Can you work these out from the model? Positions are in its coordinate system, mm. Give positions to 0.01 mm unless a question says otherwise; leave off trailing zeros. Order: outer loops, then holes, each group sorted by start corner. A loop starts at its lowest first (then second) coordinate and runs counter-clockwise, first axis right, second up. Notation, with made-up numbers: (60.5, -23.75) - (74.5, -23.75) arc R11 ccw to (74.5, -8.75) - close; hole circle Ø11 at (26, 40.5). An arc over 180 degrees is marked (long way). Answer as a JSON object with one key per item and string values.
Autodesk Inventor part; units mm, degrees
ref_plane "YZ Plane" through (0, 0, 0) normal (1, 0, 0) x (0, 1, 0)
ref_plane "XZ Plane" through (0, 0, 0) normal (0, 1, 0) x (-1, 0, 0)
ref_plane "XY Plane" through (0, 0, 0) normal (0, 0, 1) x (1, 0, 0)
sketch "Sketch1" plane through (0, 0, 0) normal (1, 0, 0) x (0, 1, 0)
  circle A0 centre (0, 0) radius 20
  line L0 (-19.9583, 1.2905) -> (-23.3333, -50.9073)
  line L1 (19.9583, 1.2905) -> (23.3333, -50.9073)
  line L2 (9.9593, -5.75) -> (0, 0) construction
  line L3 (0, -48.5721) -> (0, 22.5) construction
  arc A1 (-23.0554, -46.6095) -> (23.0554, -46.6095) centre (0, 0) ccw
  arc A2 (-23.3333, -50.9073) -> (23.3333, -50.9073) centre (0, 0) ccw
  line L4 (0, 0) -> (-23.3333, -50.9073) construction
  point P0 (0, 11.4686)
  point P1 (0, 11.4686)
  dimension "d0" = 40
  dimension "d8" = 104
  dimension "d9" = 112
  dimension "d10" = 24.624
extrude "Extrusion1" add sketch "Sketch1" along normal blind 6
extrude "Extrusion2" add sketch "Sketch1" against normal blind 47.5 from surface at 0 contours L1 A2 L0 A1
sketch "Sketch2" plane through (0, 0, 0) normal (0, 0, 1) x (1, 0, 0)
  line L0 (6, -19.9583) -> (6, 19.9583) construction
  line L1 (6, 0) -> (-47.5, 0) construction
  line L2 (-47.5, 23.3333) -> (-47.5, -23.3333)
  circle A0 centre (-20, 0) radius 23.3333
  line L3 (6, 23.3333) -> (-47.5, 23.3333)
  line L4 (-47.5, -23.3333) -> (6, -23.3333)
  line L5 (-20, 23.3333) -> (-20, -23.3333) construction
  point P0 (0, 0)
  dimension "d21" = 27.5
extrude "Extrusion3" cut sketch "Sketch2" against normal through all contours L3 A0 L4 L2
properties part number "shank_connector"
Q1. I need wall thicknesses on L1, parallel to X at y = -8.5, z = 1.5; L2, parallel to Z at x = -10, y = 0.5; L3, parallel to Z at x = -17, y = -9. Which ranges of each line are inside material? Lowest first, please.
Recorded:
{"L1": "x = 0 to 6", "L2": "z = -56 to -52", "L3": "z = -55.27 to -51.22"}
Q2. If we section it at B-B, the plane x = -7.5: Please give me the cut outline in (y, z), then the cut area to 3 significant figures.
Recorded:
{"outline": "(-23.33, -50.91) arc R56 ccw to (23.33, -50.91) - (23.06, -46.61) arc R52 cw to (-23.06, -46.61) - close", "area": "192 mm^2"}
Q3. If we section it at D-D, the plane y = 17.5: Please give me the cut outline in (x, z).
Recorded:
{"outline": "(-35.43, -53.2) - (6, -53.2) - (6, 9.68) - (0, 9.68) - (0, -48.97) - (-35.43, -48.97) - close"}
Q4. I'm going to push flat-ended pins straight in: pin 1 Ø1.5 at (x, y) = (-8.5, 3) entering from +Z; pin 2 Ø10 at (y, z) = (12.5, -28.5) entering from -X; pin 3 Ø6 at (x, y) = (-34.5, 4.5) entering from -Z. Where does each tip first touch, or does it pass through?
Recorded:
{"pin 1": "stops at z = -51.86", "pin 2": "stops at x = 0", "pin 3": "stops at z = -55.98"}
Q5. We'd pull the mould along Y, two halves only. Please class faces 1 (the face through (-43.328, 0.513, -52.284)), 2 (the face through (-21, 0, -52)), 3 (the face through (1.137, 22.013, -30.486)): released by +Y, released by -Y, zero draft, split by the parting line, or undercut.
Recorded:
{"face 1": "split by the parting line", "face 2": "undercut", "face 3": "released by +Y"}
Q6. If we section it at A-A, the plane y = 0: Please give me the cut outline in (x, z), then the cut area to 3 significant figures.
Recorded:
{"outline": "(-43.33, -56) - (6, -56) - (6, 20) - (0, 20) - (0, -52) - (-43.33, -52) - close", "area": "629 mm^2"}
Q7. If we section it at C-C, the plane z = -2: Please give me the cut outline in (x, y).
Recorded:
{"outline": "(0, -20.17) - (6, -20.17) - (6, 20.17) - (0, 20.17) - close"}
